```python
from build123d import *

# Parameters (mm, degrees)
SKETCH1_W           = 63.5
SKETCH1_H           = 152.4
BOSS_EXTRUDE1_DEPTH = 3.175
SKETCH2_R           = 1.5875
SKETCH2_R_2         = 1.190625
CUT_EXTRUDE1_DEPTH  = 159.781746826
SKETCH3_R           = 1.190625
CUT_EXTRUDE2_DEPTH  = 159.781746826


with BuildPart() as part:
    # Sketch1 → Boss-Extrude1 (new body)
    with BuildSketch(Plane(origin=(0, 0, 0), x_dir=(1, 0, 0), z_dir=(0, 1, 0))):
        Polygon((-111.686526805, 95.25), (-127, 83.918625912), (-127, -83.918625912), (-111.686526805, -95.25), (111.686526805, -95.25), (127, -83.918625912), (127, 83.918625912), (111.686526805, 95.25), align=None)
        Polygon((-107.95, -41.010963508), (-107.95, 41.010963508), (-95.25, 41.010963508), (-79.936526805, 52.342337595), (-79.936526805, 76.2), (-38.1, 76.2), (-38.1, -76.2), (-79.936526805, -76.2), (-79.936526805, -52.342337595), (-95.25, -41.010963508), align=None, mode=Mode.SUBTRACT)
        Rectangle(SKETCH1_W, SKETCH1_H, mode=Mode.SUBTRACT)
        Polygon((79.936526805, -76.2), (38.1, -76.2), (38.1, 76.2), (79.936526805, 76.2), (79.936526805, 52.342337595), (95.25, 41.010963508), (107.95, 41.010963508), (107.95, -41.010963508), (95.25, -41.010963508), (79.936526805, -52.342337595), align=None, mode=Mode.SUBTRACT)
    extrude(amount=BOSS_EXTRUDE1_DEPTH)

    # Sketch2 → Cut-Extrude1 (cut, through all)
    with BuildSketch(Plane(origin=(0, 3.175, 0), x_dir=(1, 0, 0), z_dir=(0, 1, 0))):
        with Locations(Location((-95.147512794, 56.885632681, 0), (0, 0, 270))):
            Circle(SKETCH2_R)
        with Locations(Location((-110.256011578, 77.303596941, 0), (0, 0, 270))):
            Circle(SKETCH2_R)
        with Locations(Location((110.256011578, 77.303596941, 0), (0, 0, 90))):
            Circle(SKETCH2_R)
        with Locations(Location((95.147512794, 56.885632681, 0), (0, 0, 90))):
            Circle(SKETCH2_R)
        with Locations(Location((110.256011578, -77.303596941, 0), (0, 0, 270))):
            Circle(SKETCH2_R)
        with Locations(Location((95.147512794, -56.885632681, 0), (0, 0, 270))):
            Circle(SKETCH2_R)
        with Locations(Location((-110.256011578, -77.303596941, 0), (0, 0, 90))):
            Circle(SKETCH2_R)
        with Locations(Location((-95.147512794, -56.885632681, 0), (0, 0, 90))):
            Circle(SKETCH2_R)
        with Locations(Location((-88.154790208, 79.461855841, 0), (0, 0, 270))):
            Circle(SKETCH2_R_2)
        with Locations(Location((-118.781736597, 56.799107666, 0), (0, 0, 90))):
            Circle(SKETCH2_R_2)
        with Locations(Location((118.781736597, 56.799107666, 0), (0, 0, 270))):
            Circle(SKETCH2_R_2)
        with Locations(Location((88.154790208, 79.461855841, 0), (0, 0, 90))):
            Circle(SKETCH2_R_2)
        with Locations(Location((118.781736597, -56.799107666, 0), (0, 0, 90))):
            Circle(SKETCH2_R_2)
        with Locations(Location((88.154790208, -79.461855841, 0), (0, 0, 270))):
            Circle(SKETCH2_R_2)
        with Locations(Location((-88.154790208, -79.461855841, 0), (0, 0, 90))):
            Circle(SKETCH2_R_2)
        with Locations(Location((-118.781736597, -56.799107666, 0), (0, 0, 270))):
            Circle(SKETCH2_R_2)
    extrude(amount=-CUT_EXTRUDE1_DEPTH, mode=Mode.SUBTRACT)

    # Sketch3 → Cut-Extrude2 (cut, through all)
    with BuildSketch(Plane(origin=(0, 3.175, 0), x_dir=(1, 0, 0), z_dir=(0, 1, 0))):
        with Locations(Location((-76.2, 85.725, 0), (0, 0, 270))):
            Circle(SKETCH3_R)
        with Locations(Location((-25.4, 85.725, 0), (0, 0, 270))):
            Circle(SKETCH3_R)
        with Locations(Location((25.4, 85.725, 0), (0, 0, 270))):
            Circle(SKETCH3_R)
        with Locations(Location((76.2, 85.725, 0), (0, 0, 270))):
            Circle(SKETCH3_R)
        with Locations(Location((76.2, -85.725, 0), (0, 0, 90))):
            Circle(SKETCH3_R)
        with Locations(Location((25.4, -85.725, 0), (0, 0, 90))):
            Circle(SKETCH3_R)
        with Locations(Location((-25.4, -85.725, 0), (0, 0, 90))):
            Circle(SKETCH3_R)
        with Locations(Location((-76.2, -85.725, 0), (0, 0, 90))):
            Circle(SKETCH3_R)
        with Locations(Location((-117.475, -25.4, 0), (0, 0, 270))):
            Circle(SKETCH3_R)
        with Locations(Location((-117.475, 25.4, 0), (0, 0, 270))):
            Circle(SKETCH3_R)
        with Locations(Location((117.475, 25.4, 0), (0, 0, 90))):
            Circle(SKETCH3_R)
        with Locations(Location((117.475, -25.4, 0), (0, 0, 90))):
            Circle(SKETCH3_R)
    extrude(amount=-CUT_EXTRUDE2_DEPTH, mode=Mode.SUBTRACT)


solid = part.part
```
Verification items for the finished model (mm, model axes). A direction names the side the tool comes from. Give positions to 0.01 mm unless a question says otherwise; leave off trailing zeros. Loops run counter-clockwise (first coordinate to the right, second up) from the corner with the lowest first, then second, coordinate; pieces in that order, holes last. Notation, with made-up numbers: M 85.5,16 L 113.5,16 A31 ccw 113.5,52 Z; hole C 30.5,88 d10. An arc over 180 degrees is marked long. Return JSON: item names as keys, results as strings.
1) Section check B-B, the plane x = -20.5. Enter the section's corners in (y, z) (3 decimals).
Findings:
{"outline": "M 0,-95.25 L 3.175,-95.25 L 3.175,-76.2 L 0,-76.2 Z; M 0,76.2 L 3.175,76.2 L 3.175,95.25 L 0,95.25 Z"}
2) Tool access check on faces 1 (the flat face through (-119.45, 1.565, 89.505)), 2 (the flat face through (87.486, 1.565, -46.756)). Record the directions out of +Z, -Z, +X, -X, +Y, -Y that give a thin tool (end or side, any length) a straight path to the whole face; none if there is none.
Findings:
{"face 1": "+Z, -X, +Y, -Y", "face 2": "+Y, -Y"}
3) Material ranges on L1, parallel to X at y = 0.7, z = -25.5; L2, parallel to X at y = 0.65, z = 14; L3, parallel to X at y = 0.5, z = 74, recorded low to high. Write a range as [from, to].
Findings:
{"L1": "x = [-127, -118.66], [-116.29, -107.95], [-38.1, -31.75], [31.75, 38.1], [107.95, 116.29], [118.66, 127]", "L2": "x = [-127, -107.95], [-38.1, -31.75], [31.75, 38.1], [107.95, 127]", "L3": "x = [-127, -79.94], [-38.1, -31.75], [31.75, 38.1], [79.94, 127]"}
4) Section check D-D, the plane y = 1.05. Count the separate pieces of the cut face and the enclosed holes in it, and give its area (3 significant figures).
Findings:
{"separate pieces": "1", "enclosed holes": "31", "area": "20,500 mm2"}
5) Mould release check, pull along Z, two halves, no side actions. Record for faces 3 (the flat face through (-119.24, 1.57, -89.66)), 4 (the flat face through (-2, 3.175, 83)), 5 (the flat face through (-87.486, 1.565, 46.756)), 6 (the flat face through (119.24, 1.57, 89.66)): released by +Z, released by -Z, zero draft, split by the parting line, or undercut.
Findings:
{"face 3": "released by -Z", "face 4": "zero draft", "face 5": "undercut", "face 6": "released by +Z"}
6) Section check A-A, the plane z = -36.5. Enter the section's corners in (x, y) (3 decimals), and give its area (3 significant figures).
Findings:
{"outline": "M -127,0 L -107.95,0 L -107.95,3.175 L -127,3.175 Z; M -38.1,0 L -31.75,0 L -31.75,3.175 L -38.1,3.175 Z; M 31.75,0 L 38.1,0 L 38.1,3.175 L 31.75,3.175 Z; M 107.95,0 L 127,0 L 127,3.175 L 107.95,3.175 Z", "area": "161 mm2"}
7) Section check C-C, the plane z = -66. Enter the section's corners in (x, y) (3 decimals).
Findings:
{"outline": "M -127,0 L -79.937,0 L -79.937,3.175 L -127,3.175 Z; M -38.1,0 L -31.75,0 L -31.75,3.175 L -38.1,3.175 Z; M 31.75,0 L 38.1,0 L 38.1,3.175 L 31.75,3.175 Z; M 79.937,0 L 127,0 L 127,3.175 L 79.937,3.175 Z"}
